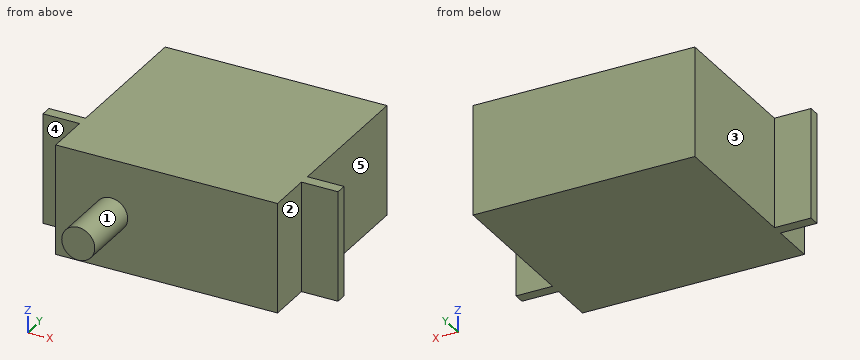
```python
from build123d import *

# Parameters (mm, degrees)
F0_W     = 40.3
F0_H     = 20
F1_DEPTH = 36.6
F3_W     = 6.65
F3_H     = 20
F4_DEPTH = 2
F6_R     = 3
F7_DEPTH = 11


with BuildPart() as f1:
    # F0 (on Front) → F1 (new body)
    with BuildSketch(Plane.XZ):
        Rectangle(F0_W, F0_H)
    extrude(amount=-F1_DEPTH)

    # F3 (on offset) → F4 (join)
    with BuildSketch(Plane(origin=(0, 10, 0), x_dir=(-1, 0, 0), z_dir=(0, 1, 0))):
        with Locations((-23.475, 0)):
            Rectangle(F3_W, F3_H)
        with Locations((23.475, 0)):
            Rectangle(F3_W, F3_H)
    extrude(amount=-F4_DEPTH)

    # F6 (on offset) → F7 (join, through all)
    with BuildSketch(Plane(origin=(0, -11, 0), x_dir=(-1, 0, 0), z_dir=(0, 1, 0))):
        with Locations((10.075, 0)):
            Circle(F6_R)
    extrude(amount=F7_DEPTH)


solid = f1.part
```
Work out the finished part from the listing and answer in its coordinate system (mm). Face numbers are marked on the shaded views. A direction names the side the tool comes from. Give positions to 0.01 mm unless a question says otherwise; leave off trailing zeros. Loops run counter-clockwise (first coordinate to the right, second up) from the corner with the lowest first, then second, coordinate; pieces in that order, holes last. Notation, with made-up numbers: (0.25, -19.75) - (6.25, -19.75) arc R18 cw to (6.25, -8.75) - close; hole circle Ø11 at (-37.5, -7.5). An arc over 180 degrees is marked (long way). Use CSV: the item, a comma, the result in double quotes. Start each with the question number.
(1) Each of these flat-tipped pins is pushed along its axis until it touches: pin 1 (2.5 mm diameter, centred on y = 4, z = 4, fed in from -X); pin 2 (5.5 mm diameter, centred on x = -23.5, z = -0.5, fed in from -Y); pin 3 (6 mm diameter, centred on y = 31, z = -6.5, fed in from -X); pin 4 (6 mm diameter, centred on y = 7, z = -5, fed in from +X). Where does it stop, or does it pass through?
(2) Find the intervals of material crossed by L1, parallel to Y at x = -13.5, z = 5; L2, parallel to X at y = 21.5, z = 0.75; L3, parallel to Y at x = 20.5, z = 5.5, in increasing order.
(3) Find section C-C, the plane y = 28. Determine the outline of the cut face in (x, z), plus the area to 3 significant figures.
(4) A tool of negligible diameter and unlimited length cuts with its end or side. For the marked faces 1, 2, 3, 4 and 5, from which of +Z, -Z, +X, -X, +Y, -Y can it reach the whole face along a straight path? Write none if from no direction.
(5) Find section A-A, the plane z = 0. Determine the outline of the cut face in (x, y) (3 decimals).
(6) Find section B-B, the plane x = 1.5. Determine the outline of the cut face in (y, z).
Results found:
1,pin 1,"x = -20.15"
1,pin 2,"y = 8"
1,pin 3,"x = -20.15"
1,pin 4,"x = 26.8"
2,L1,"0 to 36.6"
2,L2,"-20.15 to 20.15"
2,L3,"8 to 10"
3,outline,"(-20.15, -10) - (20.15, -10) - (20.15, 10) - (-20.15, 10) - close"
3,area,"806 mm^2"
4,face 1,"-Y"
4,face 2,"+Z, -Z, +X, -Y"
4,face 3,"+Z, -Z, -X, +Y"
4,face 4,"+Z, -Z, -X, -Y"
4,face 5,"+Z, -Z, +X, +Y"
5,outline,"(-26.8, 8) - (-20.15, 8) - (-20.15, 0) - (-13.075, 0) - (-13.075, -11) - (-7.075, -11) - (-7.075, 0) - (20.15, 0) - (20.15, 8) - (26.8, 8) - (26.8, 10) - (20.15, 10) - (20.15, 36.6) - (-20.15, 36.6) - (-20.15, 10) - (-26.8, 10) - close"
6,outline,"(0, -10) - (36.6, -10) - (36.6, 10) - (0, 10) - close"
